Build history of the part. All positions in model axes, mm. Face numbers are marked on the shaded views. A direction names the side the tool comes from. Give positions to 0.01 mm unless a question says otherwise; leave off trailing zeros. Write each loop counter-clockwise with the first axis right and the second up, starting at its lowest first coordinate (ties: lowest second). Pieces come first, ordered by that corner, then holes. Notation, with made-up numbers: M -5.75,-8 L 3.25,-8 A17 ccw 3.25,7 Z; hole C 38,15 d5. An arc over 180 degrees is marked long. Return JSON: item names as keys, results as strings. Group by question number.
Q1. Wall check: probe 1 along Y at (x, z) = (9.25, 6); probe 2 along Y at (x, z) = (15.15, 10); probe 3 along X at (y, z) = (6.5, 45). Give the ranges that are in metal, low to high.
Q2. Band-saw the part on B-B, the plane x = 5. Give the cut face in (y, z).
Q3. Band-saw the part on D-D, the plane x = 11.25. Give the cut face in (y, z).
Q4. Pull direction Y, two halves, no side cores. Call the marked faces 3, 4, 5 and 6: +Y half, -Y half, draft (parallel to the pull), parting line (faces both ways), or undercut.
Q5. Band-saw the part on A-A, the plane y = 6.5. Count the separate pieces of the cut face and the enclosed holes in it, then the cut area to 3 significant figures.
Q6. Band-saw the part on C-C, the plane z = 93.9. Give the cut face in (x, y).
Q7. Tool access for the marked faces 1 and 2: list every direction of +Z, -Z, +X, -X, +Y, -Y with a clear straight run to the whole face (end or side of a thin tool).
Q8. Flat gauge pins, fed straight in: pin 1 Ø1 at (y, z) = (9.5, 68) entering from -X; pin 2 Ø4 at (y, z) = (7, 95) entering from -X; pin 3 Ø1 at (x, y) = (11, 9) entering from +Z. Where does each tip first touch, or does it go through?
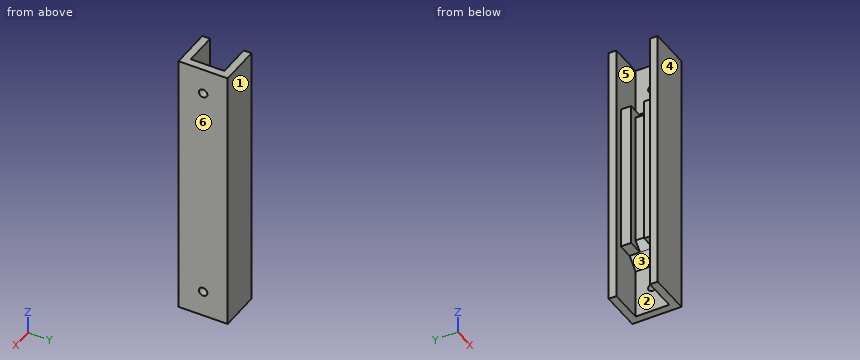
from build123d import *

# Parameters (mm, degrees)
SKETCH_1_W          = 19
SKETCH_1_H          = 19
SKETCH_1_W_2        = 13
SKETCH_1_H_2        = 13
EXTRUDE_1_DEPTH     = 103.9
SKETCH_2_R          = 1.65
CUT_EXTRUDE_1_DEPTH = 30
SKETCH_3_W          = 116.915177823
SKETCH_3_H          = 46.219516436
CUT_EXTRUDE_2_DEPTH = 3
SKETCH_4_W          = 5
SKETCH_4_H          = 13
EXTRUDE_1_2_DEPTH   = 10
SKETCH_5_W          = 47.9
SKETCH_5_H          = 5
EXTRUDE_2_DEPTH     = 10
SKETCH_6_W          = 57.9
SKETCH_6_H          = 13
EXTRUDE_3_DEPTH     = 10
SKETCH_8_W          = 57.9
SKETCH_8_H          = 5
CUT_EXTRUDE_3_DEPTH = 3
CHAMFER_1_SIZE      = 3
CHAMFER_2_SIZE      = 4


with BuildPart() as part:
    # 草图1 → Extrude 1 (new body)
    with BuildSketch(Plane.XY):
        with Locations((6.5, 6.5)):
            Rectangle(SKETCH_1_W, SKETCH_1_H)
        with Locations((6.5, 6.5)):
            Rectangle(SKETCH_1_W_2, SKETCH_1_H_2, mode=Mode.SUBTRACT)
    extrude(amount=EXTRUDE_1_DEPTH)

    # 草图2 → 切除-拉伸1 (cut)
    with BuildSketch(Plane.ZY.offset(3)):
        with Locations((10, 6.5)):
            Circle(SKETCH_2_R)
        with Locations((93.9, 6.5)):
            Circle(SKETCH_2_R)
    extrude(amount=-CUT_EXTRUDE_1_DEPTH, mode=Mode.SUBTRACT)

    # 草图3 → 切除-拉伸2 (cut)
    with BuildSketch(Plane.ZY.offset(3)):
        with Locations((53.162237228, 0.202739406)):
            Rectangle(SKETCH_3_W, SKETCH_3_H)
    extrude(amount=-CUT_EXTRUDE_2_DEPTH, mode=Mode.SUBTRACT)

    # 草图4 → Extrude 1 2 (add)
    with BuildSketch(Plane.ZY.offset(-13)):
        with Locations((25.5, 6.5)):
            Rectangle(SKETCH_4_W, SKETCH_4_H)
        with Locations((78.4, 6.5)):
            Rectangle(SKETCH_4_W, SKETCH_4_H)
    extrude(amount=EXTRUDE_1_2_DEPTH)

    # 草图5 → 凸台-拉伸2 (add)
    with BuildSketch(Plane.ZY.offset(-13)):
        with Locations((51.95, 6.5)):
            Rectangle(SKETCH_5_W, SKETCH_5_H)
    extrude(amount=EXTRUDE_2_DEPTH)

    # 草图6 → 凸台-拉伸3 (add)
    with BuildSketch(Plane.ZY.offset(-13)):
        with Locations((51.95, 6.5)):
            Rectangle(SKETCH_6_W, SKETCH_6_H)
    extrude(amount=EXTRUDE_3_DEPTH)

    # 草图8 → 切除-拉伸3 (cut)
    with BuildSketch(Plane.ZY.offset(-3)):
        with Locations((51.95, 6.5)):
            Rectangle(SKETCH_8_W, SKETCH_8_H)
    extrude(amount=-CUT_EXTRUDE_3_DEPTH, mode=Mode.SUBTRACT)

    # 倒角1
    chamfer_1_edges = [part.edges().sort_by_distance(p)[0] for p in [
        (6, 6.5, 23),
        (6, 6.5, 80.9),
    ]]
    chamfer(chamfer_1_edges, length=CHAMFER_1_SIZE)

    # 倒角2
    chamfer_2_edges = [part.edges().sort_by_distance(p)[0] for p in [
        (13, 6.5, 23),
        (13, 6.5, 80.9),
    ]]
    chamfer(chamfer_2_edges, length=CHAMFER_2_SIZE - 0.0001)  # a hair under: the kernel refuses the full size


solid = part.part
From the geometry:
{
 "1": {"probe 1": "y = -3 to 0, 13 to 16", "probe 2": "y = -3 to 4.85, 8.15 to 16", "probe 3": "x = 6 to 16"},
 "2": {"outline": "M -3,0 L 0,0 L 0,23 L 4,23 L 4,80.9 L 0,80.9 L 0,103.9 L -3,103.9 Z; M 9,23 L 13,23 L 13,0 L 16,0 L 16,103.9 L 13,103.9 L 13,80.9 L 9,80.9 Z"},
 "3": {"outline": "M -3,0 L 0,0 L 0,20.75 L 13,20.75 L 13,0 L 16,0 L 16,103.9 L 13,103.9 L 13,83.15 L 0,83.15 L 0,103.9 L -3,103.9 Z"},
 "4": {"face 3": "undercut", "face 4": "-Y half", "face 5": "undercut", "face 6": "draft"},
 "5": {"separate pieces": "3", "enclosed holes": "0", "area": "704 mm^2"},
 "6": {"outline": "M 0,-3 L 16,-3 L 16,4.85 L 13,4.85 L 13,0 L 0,0 Z; M 0,13 L 13,13 L 13,8.15 L 16,8.15 L 16,16 L 0,16 Z"},
 "7": {"face 1": "+Z, -Z, +X, -X, +Y", "face 2": "-Z, -X"},
 "8": {"pin 1": "stops at x = 3", "pin 2": "stops at x = 13", "pin 3": "stops at z = 83.4"}
}
